Source: CAD feature listing. Evaluate the final solid. Frame: model axes, mm. Round coordinates to 2 decimals unless told otherwise and drop trailing zeros. Order: outer loops, then holes, each group sorted by start corner. A loop starts at its lowest first (then second) coordinate and runs counter-clockwise, first axis right, second up. Notation, with made-up numbers: M 64.25,87 L 104.25,87 A26 cw 104.25,124 Z; hole C 64.5,37 d8. An arc over 180 degrees is marked long. Use CSV: the item, a comma, the result in double quotes. Start each with the question number.
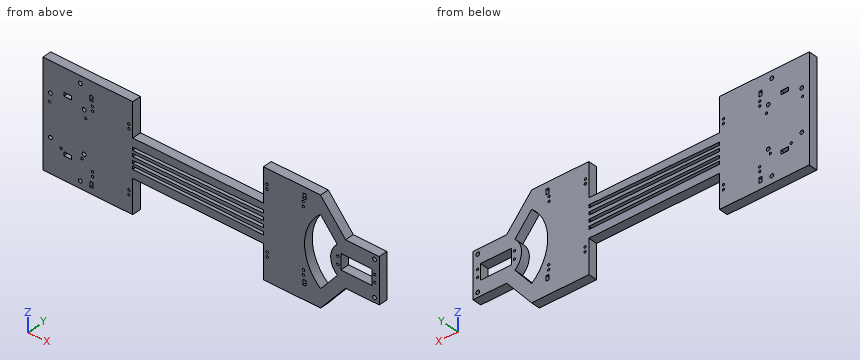
```python
from build123d import *

# Parameters (mm, degrees)
SKETCH1_R           = 1.5
SKETCH1_R_2         = 2.5
SKETCH1_W           = 10
SKETCH1_H           = 5
SKETCH1_W_2         = 4
SKETCH1_H_2         = 7
SKETCH1_W_3         = 41.5
SKETCH1_H_3         = 20.5
BOSS_EXTRUDE1_DEPTH = 12
SKETCH2_R           = 2.5
CUT_EXTRUDE1_DEPTH  = 13


with BuildPart() as part:
    # Sketch1 → Boss-Extrude1 (new body)
    with BuildSketch(Plane(origin=(0, 0, 0), x_dir=(1, 0, 0), z_dir=(0, 1, 0))):
        Polygon((295, 140), (450, 140), (450, 0), (295, 0), (295, 45), (120, 45), (120, 0), (0, 0), (0, 140), (120, 140), (120, 95), (295, 95), align=None)
        with Locations(Location((8.95, 51, 0), (0, 0, 270))):  # turned: the seam where the file's is
            Circle(SKETCH1_R, mode=Mode.SUBTRACT)
        with Locations(Location((57.15, 49.7, 0), (0, 0, 270))):  # turned: the seam where the file's is
            Circle(SKETCH1_R, mode=Mode.SUBTRACT)
        with Locations(Location((24.15, 101.8, 0), (0, 0, 270))):  # turned: the seam where the file's is
            Circle(SKETCH1_R, mode=Mode.SUBTRACT)
        with Locations(Location((52.05, 101.8, 0), (0, 0, 270))):  # turned: the seam where the file's is
            Circle(SKETCH1_R, mode=Mode.SUBTRACT)
        with Locations(Location((50, 130.475, 0), (0, 0, 270))):  # turned: the seam where the file's is
            Circle(SKETCH1_R_2, mode=Mode.SUBTRACT)
        with Locations(Location((50, 9.525, 0), (0, 0, 270))):  # turned: the seam where the file's is
            Circle(SKETCH1_R_2, mode=Mode.SUBTRACT)
        with Locations(Location((10, 95, 0), (0, 0, 270))):  # turned: the seam where the file's is
            Circle(SKETCH1_R_2, mode=Mode.SUBTRACT)
        with Locations(Location((10, 40, 0), (0, 0, 270))):  # turned: the seam where the file's is
            Circle(SKETCH1_R_2, mode=Mode.SUBTRACT)
        with Locations(Location((55, 40, 0), (0, 0, 270))):  # turned: the seam where the file's is
            Circle(SKETCH1_R_2, mode=Mode.SUBTRACT)
        with Locations(Location((55, 95, 0), (0, 0, 270))):  # turned: the seam where the file's is
            Circle(SKETCH1_R_2, mode=Mode.SUBTRACT)
        with Locations(Location((394.5, 75, 0), (0, 0, 270))):  # turned: the seam where the file's is
            Circle(SKETCH1_R, mode=Mode.SUBTRACT)
        with Locations(Location((394.5, 65, 0), (0, 0, 270))):  # turned: the seam where the file's is
            Circle(SKETCH1_R, mode=Mode.SUBTRACT)
        with Locations(Location((444, 75, 0), (0, 0, 270))):  # turned: the seam where the file's is
            Circle(SKETCH1_R, mode=Mode.SUBTRACT)
        with Locations(Location((444, 65, 0), (0, 0, 270))):  # turned: the seam where the file's is
            Circle(SKETCH1_R, mode=Mode.SUBTRACT)
        with Locations(Location((114.940849733, 111.822591207, 0), (0, 0, 270))):  # turned: the seam where the file's is
            Circle(SKETCH1_R, mode=Mode.SUBTRACT)
        with Locations(Location((114.919764018, 117.822591207, 0), (0, 0, 270))):  # turned: the seam where the file's is
            Circle(SKETCH1_R, mode=Mode.SUBTRACT)
        with Locations(Location((66.34114984, 111.651797976, 0), (0, 0, 270))):  # turned: the seam where the file's is
            Circle(SKETCH1_R, mode=Mode.SUBTRACT)
        with Locations(Location((66.320064126, 117.651797976, 0), (0, 0, 270))):  # turned: the seam where the file's is
            Circle(SKETCH1_R, mode=Mode.SUBTRACT)
        with Locations(Location((114.91898341, 36.133817731, 0), (0, 0, 270))):  # turned: the seam where the file's is
            Circle(SKETCH1_R, mode=Mode.SUBTRACT)
        with Locations(Location((114.864297696, 30.133817731, 0), (0, 0, 270))):  # turned: the seam where the file's is
            Circle(SKETCH1_R, mode=Mode.SUBTRACT)
        with Locations(Location((66.266327532, 30.577999595, 0), (0, 0, 270))):  # turned: the seam where the file's is
            Circle(SKETCH1_R, mode=Mode.SUBTRACT)
        with Locations(Location((66.321013247, 36.577999595, 0), (0, 0, 270))):  # turned: the seam where the file's is
            Circle(SKETCH1_R, mode=Mode.SUBTRACT)
        with Locations(Location((300.048791832, 103.567263833, 0), (0, 0, 270))):  # turned: the seam where the file's is
            Circle(SKETCH1_R, mode=Mode.SUBTRACT)
        with Locations(Location((300.082906118, 109.567263833, 0), (0, 0, 270))):  # turned: the seam where the file's is
            Circle(SKETCH1_R, mode=Mode.SUBTRACT)
        with Locations(Location((348.682120582, 109.290942585, 0), (0, 0, 270))):  # turned: the seam where the file's is
            Circle(SKETCH1_R, mode=Mode.SUBTRACT)
        with Locations(Location((348.648006297, 103.290942585, 0), (0, 0, 270))):  # turned: the seam where the file's is
            Circle(SKETCH1_R, mode=Mode.SUBTRACT)
        with Locations(Location((299.691143962, 25.55274586, 0), (0, 0, 270))):  # turned: the seam where the file's is
            Circle(SKETCH1_R, mode=Mode.SUBTRACT)
        with Locations(Location((299.595658248, 19.55274586, 0), (0, 0, 270))):  # turned: the seam where the file's is
            Circle(SKETCH1_R, mode=Mode.SUBTRACT)
        with Locations(Location((348.284990804, 24.779409497, 0), (0, 0, 270))):  # turned: the seam where the file's is
            Circle(SKETCH1_R, mode=Mode.SUBTRACT)
        with Locations(Location((348.18950509, 18.779409497, 0), (0, 0, 270))):  # turned: the seam where the file's is
            Circle(SKETCH1_R, mode=Mode.SUBTRACT)
        Polygon((120, 83.84), (295, 84.455), (295, 80.455), (120, 79.84), align=None, mode=Mode.SUBTRACT)
        Polygon((120, 76.59), (295, 75.595), (295, 71.595), (120, 72.59), align=None, mode=Mode.SUBTRACT)
        Polygon((120, 68.09), (295, 66.495), (295, 62.495), (120, 64.09), align=None, mode=Mode.SUBTRACT)
        Polygon((120, 60.42), (295, 57.635), (295, 53.635), (120, 56.42), align=None, mode=Mode.SUBTRACT)
        with Locations((33, 106.8)):
            Rectangle(SKETCH1_W, SKETCH1_H, mode=Mode.SUBTRACT)
        with Locations((33, 33.2)):
            Rectangle(SKETCH1_W, SKETCH1_H, mode=Mode.SUBTRACT)
        with Locations((65, 128.5)):
            Rectangle(SKETCH1_W_2, SKETCH1_H_2, mode=Mode.SUBTRACT)
        with Locations((65, 21.5)):
            Rectangle(SKETCH1_W_2, SKETCH1_H_2, mode=Mode.SUBTRACT)
        with Locations((419.25, 70)):
            Rectangle(SKETCH1_W_3, SKETCH1_H_3, mode=Mode.SUBTRACT)
        with BuildLine():
            Line((393.930309758, 50.848888922), (371.432743419, 24.037333413))
            ThreePointArc((371.432743419, 24.037333413), (350, 70), (371.432743419, 115.962666587))
            Line((371.432743419, 115.962666587), (393.930309758, 89.151111078))
            ThreePointArc((393.930309758, 89.151111078), (385, 70), (393.930309758, 50.848888922))
        make_face(mode=Mode.SUBTRACT)
        with Locations((350, 118.5)):
            Rectangle(SKETCH1_W_2, SKETCH1_H_2, mode=Mode.SUBTRACT)
        with Locations((350, 11.5)):
            Rectangle(SKETCH1_W_2, SKETCH1_H_2, mode=Mode.SUBTRACT)
    extrude(amount=BOSS_EXTRUDE1_DEPTH)

    # Sketch2 → Cut-Extrude1 (cut, through all)
    with BuildSketch(Plane(origin=(0, 12, 0), x_dir=(1, 0, 0), z_dir=(0, 1, 0))):
        with Locations(Location((443.65, 93.65, 0), (0, 0, 270))):  # turned: the seam where the file's is
            Circle(SKETCH2_R)
        with Locations(Location((443.65, 46.35, 0), (0, 0, 270))):  # turned: the seam where the file's is
            Circle(SKETCH2_R)
        Polygon((371.432743419, 140), (404.996728666, 100), (450, 100), (450, 140), align=None)
        Polygon((371.432743419, 0), (404.996728666, 40), (450, 40), (450, 0), align=None)
    extrude(amount=-CUT_EXTRUDE1_DEPTH, mode=Mode.SUBTRACT)


solid = part.part
```
(1) Section B-B on y = 7.5. Give the number of separate pieces and of enclosed holes in the cut face, plus the area to 3 significant figures.
(2) Section A-A on x = 151. Return loops of the section in (y, z), plus the area to 3 significant figures.
(3) Line query: line 1 along X through (y, z) = (6, -71); line 2 along Z through (x, y) = (235.5, 11.75); line 3 along X through (y, z) = (7, -79.5). Output: solid intervals per line, ascending.
(4) Contact query for flat-ended pins moving along their axis: P1, Ø5, axis at x = 142.5, y = 6, coming from the +Z side; P2, Ø3.5, axis at x = 415, y = 5.5, coming from the -Z side. Output: stop coordinate, or through.
Results below:
1,separate pieces,"1"
1,enclosed holes,"44"
1,area,"35,500 mm2"
2,outline,"M 0,-95 L 12,-95 L 12,-83.95 L 0,-83.95 Z; M 0,-79.95 L 12,-79.95 L 12,-76.41 L 0,-76.41 Z; M 0,-72.41 L 12,-72.41 L 12,-67.81 L 0,-67.81 Z; M 0,-63.81 L 12,-63.81 L 12,-59.93 L 0,-59.93 Z; M 0,-55.93 L 12,-55.93 L 12,-45 L 0,-45 Z"
2,area,"408 mm2"
3,line 1,"x = 0 to 350.01, 385.02 to 398.5, 440 to 450"
3,line 2,"z = -95 to -84.25, -80.25 to -75.93, -71.93 to -67.04, -63.04 to -58.58, -54.58 to -45"
3,line 3,"x = 0 to 350.76, 386.88 to 398.5, 440 to 450"
4,P1,"stops at z = -45"
4,P2,"stops at z = -100"
